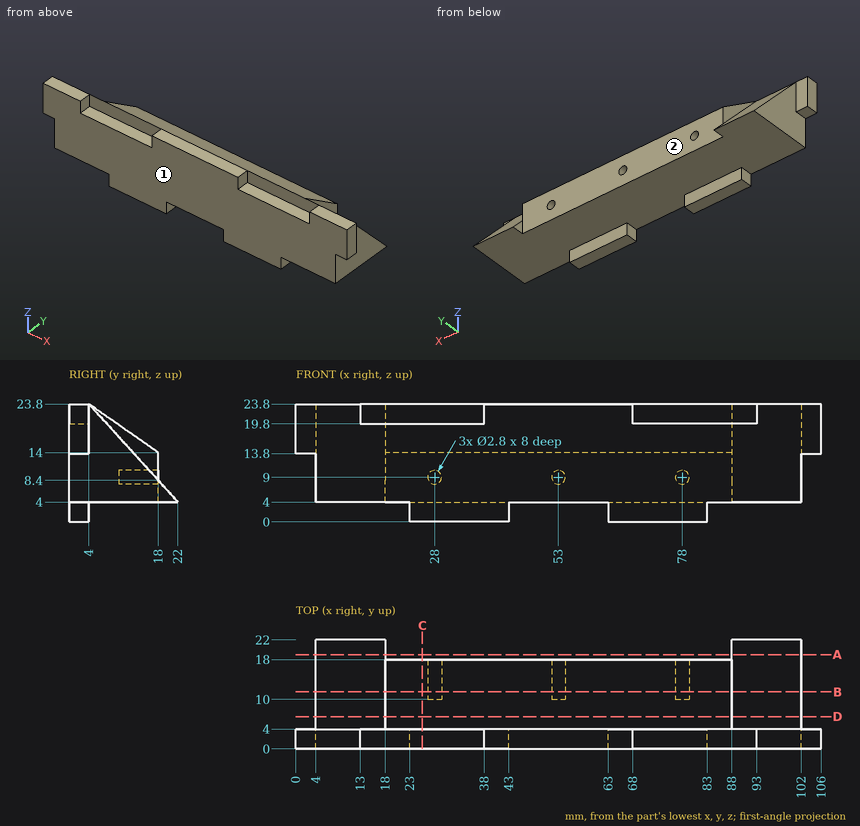
The drawing under review shows one solid part. Ordinate dimensions are in mm from its lowest x, y, z. Round coordinates to 2 decimals unless told otherwise and drop trailing zeros. Loops run counter-clockwise (first coordinate to the right, second up) from the corner with the lowest first, then second, coordinate; pieces in that order, holes last. Notation, with made-up numbers: (48, 80.25) - (105, 80.25) arc R19 ccw to (105, 86.25) - close; hole circle Ø4 at (49.5, 64.25). An arc over 180 degrees is marked (long way). Use one line per item in the form item = value.
Item 1: For line 1 (X direction, y = 13.25, z = 9); line 2 (X direction, y = 2, z = 2); line 3 (X direction, y = 11, z = 10), list the stretches that pass through material, from the lowest coordinate up.
Answers:
line_1 = 4 to 26.6, 29.4 to 51.6, 54.4 to 76.6, 79.4 to 102
line_2 = 23 to 43, 63 to 83
line_3 = 4 to 27.02, 28.98 to 52.02, 53.98 to 77.02, 78.98 to 102
Item 2: Consider section B-B on y = 11.5. Write out the cut boundary in (x, z), then the cut area to 3 significant figures.
Answers:
outline = (4, 4) - (102, 4) - (102, 15.55) - (88, 15.55) - (88, 18.55) - (18, 18.55) - (18, 15.55) - (4, 15.55) - close; hole circle Ø2.8 at (28, 9); hole circle Ø2.8 at (53, 9); hole circle Ø2.8 at (78, 9)
area = 1,320 mm^2
Item 3: Clearance check with flat-ended pins moving along their axes: P1, Ø4.5, axis at x = 104.5, z = 17.5, coming from the +Y side; P2, Ø6, axis at y = 13, z = 11, coming from the +X side; P3, Ø6, axis at x = 39, y = 13.5, coming from the -Z side. State where each tip first meets the part, or that it passes through.
Answers:
P1 = 4
P2 = 102
P3 = 4
Item 4: Consider section A-A on y = 19. Write out the cut boundary in (x, z), then the cut area to 3 significant figures.
Answers:
outline = (4, 4) - (18, 4) - (18, 7.3) - (4, 7.3) - close; (88, 4) - (102, 4) - (102, 7.3) - (88, 7.3) - close
area = 92.4 mm^2
Item 5: Consider section C-C on x = 25.5. Write out the cut boundary in (y, z).
Answers:
outline = (0, 0) - (4, 0) - (4, 4) - (18, 4) - (18, 14) - (4, 23.8) - (4, 19.8) - (0, 19.8) - close
Item 6: Mouldability with a two-part tool opening along X and no side actions: class the marked faces 1 and 2 as +X half, -X half, draft (parallel to the pull), parting line (faces both ways), or undercut.
Answers:
face_1 = draft
face_2 = undercut
Item 7: Consider section D-D on y = 6.5. Write out the cut boundary in (x, z).
Answers:
outline = (4, 4) - (102, 4) - (102, 21.05) - (88, 21.05) - (88, 22.05) - (18, 22.05) - (18, 21.05) - (4, 21.05) - close
